Geometry: final body of the model. Coordinates: model frame, mm. Face numbers are marked on the shaded views. A direction names the side the tool comes from. Coordinates: 2 decimals unless noted, no trailing zeros. Write each loop counter-clockwise with the first axis right and the second up, starting at its lowest first coordinate (ties: lowest second). Pieces come first, ordered by that corner, then holes.
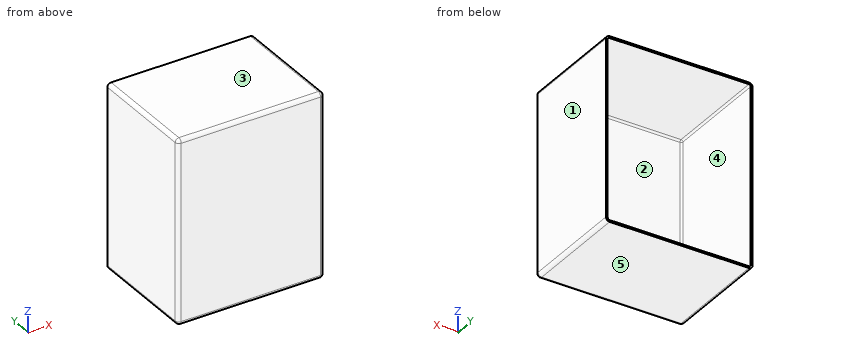
from build123d import *

# Parameters (mm, degrees)
CROQUIS1_W     = 400
CROQUIS1_H     = 500
EXTRUIR1_DEPTH = 300
REDONDEO1_R    = 10
VACIADO1_T     = -5


with BuildPart() as part:
    # Croquis1 → Extruir1 (new body)
    with BuildSketch(Plane(origin=(0, 0, 0), x_dir=(1, 0, 0), z_dir=(0, 1, 0))):
        Rectangle(CROQUIS1_W, CROQUIS1_H)
    extrude(amount=EXTRUIR1_DEPTH)

    # Redondeo1
    redondeo1_edges = [part.edges().sort_by_distance(p)[0] for p in [
        (0, 0, -250),
        (200, 0, 0),
        (0, 0, 250),
        (-200, 0, 0),
        (-200, 150, -250),
        (200, 150, -250),
        (200, 150, 250),
        (-200, 150, 250),
    ]]
    fillet(redondeo1_edges, radius=REDONDEO1_R)

    # Vaciado1
    vaciado1_openings = [part.faces().sort_by_distance(p)[0] for p in [
        (0, 300, 0),
    ]]
    offset(amount=VACIADO1_T, openings=vaciado1_openings, kind=Kind.INTERSECTION)


solid = part.part
Item 1: Section C-C, the plane x = -139.5. Output: boundary loops of the cut face in (y, z), plus the area to 3 significant figures.
Derived:
outline: (0, -240) arc R10 ccw to (10, -250) - (300, -250) - (300, -245) - (10, -245) arc R5 cw to (5, -240) - (5, 240) arc R5 cw to (10, 245) - (300, 245) - (300, 250) - (10, 250) arc R10 ccw to (0, 240) - close
area: 5,420 mm2
Item 2: Section B-B, the plane z = 49. Output: boundary loops of the cut face in (x, y), plus the area to 3 significant figures.
Derived:
outline: (-200, 10) arc R10 ccw to (-190, 0) - (190, 0) arc R10 ccw to (200, 10) - (200, 300) - (195, 300) - (195, 10) arc R5 cw to (190, 5) - (-190, 5) arc R5 cw to (-195, 10) - (-195, 300) - (-200, 300) - close
area: 4,920 mm2
Item 3: Section A-A, the plane y = 154. Output: boundary loops of the cut face in (x, z).
Derived:
outline: (-200, -240) arc R10 ccw to (-190, -250) - (190, -250) arc R10 ccw to (200, -240) - (200, 240) arc R10 ccw to (190, 250) - (-190, 250) arc R10 ccw to (-200, 240) - close; hole (-195, -240) arc R5 ccw to (-190, -245) - (190, -245) arc R5 ccw to (195, -240) - (195, 240) arc R5 ccw to (190, 245) - (-190, 245) arc R5 ccw to (-195, 240) - close
Item 4: Pull-direction query (Z, two-part tool) for the marked faces 1, 2 and 3; classes: released by +Z, released by -Z, zero draft, split by the parting line, or undercut.
Derived:
face 1: zero draft
face 2: undercut
face 3: released by +Z
Item 5: Material intervals for probe 1 along X at (y, z) = (161, 19.5); probe 2 along Z at (x, y) = (43.5, 123.5); probe 3 along Y at (x, z) = (-46.5, -159.5), sorted ascending.
Derived:
probe 1: x = -200 to -195, 195 to 200
probe 2: z = -250 to -245, 245 to 250
probe 3: y = 0 to 5
Item 6: Set-up query: the marked faces 4 and 5. Return all of +Z, -Z, +X, -X, +Y, -Y with unobstructed straight access to the full face (end or side cutting, diameter ignored); none if empty.
Derived:
face 4: +Y
face 5: -Z, +X, -X, +Y, -Y
